Here's how the part is built. I have some questions about the finished solid (model axes, mm). Round coordinates to 2 decimals unless told otherwise and drop trailing zeros. Order: outer loops, then holes, each group sorted by start corner. A loop starts at its lowest first (then second) coordinate and runs counter-clockwise, first axis right, second up. Notation, with made-up numbers: (13.25, 47.25) -> (36.25, 47.25) arc R24 cw to (36.25, 62.25) -> close; hole circle Ø6 at (65, 73.5). An arc over 180 degrees is marked (long way). Use a Markdown table: item, result. Add a question column.
(1) If I drill on probe 1 along Z at (x, y) = (-25, 6.25); probe 2 along X at (y, z) = (1.5, 0.75); probe 3 along X at (y, z) = (8, -0.5), over which ranges is the centre line in solid material (lowest first)?
(2) I want a section at B-B, the plane z = 0. Please give me the cut outline in (x, y).
(3) I want a section at A-A, the plane x = -5. Please give me the cut outline in (y, z).
(4) Thinking about a two-plate mould opening in Z: for faces 1 (the face through (-23.35, 4.93, -0.07)), 2 (the face through (-42, 0, 0)), 3 (the face through (-42, 5, -5)), which applies, pulls with the +Z half, pulls with the -Z half, needs draft (parallel to the pull), parting line crosses it, or undercut?
(5) I want a section at C-C, the plane y = 1.5. Please give me the cut outline in (x, z), then the cut area to 3 significant figures.
Autodesk Inventor part; units mm, degrees
ref_plane "YZ Plane" through (0, 0, 0) normal (1, 0, 0) x (0, 1, 0)
ref_plane "XZ Plane" through (0, 0, 0) normal (0, 1, 0) x (-1, 0, 0)
ref_plane "XY Plane" through (0, 0, 0) normal (0, 0, 1) x (1, 0, 0)
sketch "Sketch1" plane through (0, 0, 0) normal (0, 1, 0) x (-1, 0, 0)
  line L0 (85, 5) -> (0, 5)
  line L1 (0, 5) -> (0, -5)
  line L2 (0, -5) -> (85, -5)
  line L3 (85, -5) -> (85, 5)
  line L4 (25, 0) -> (5, 0) construction
  circle A0 centre (25, 0) radius 1.65
  circle A1 centre (5, 0) radius 1.65
  point P0 (0, 0)
  point P1 (0, 0)
  dimension "d0" = 10
  dimension "d1" = 20
  dimension "d2" = 3.3
  dimension "d3" = 5
  dimension "d6" = 85
extrude "Extrusion1" add sketch "Sketch1" along normal blind 10
properties part number "Tope X" material "Polypropylene"
Taken from the geometry:
| question | item | result |
|---|---|---|
| 1 | probe 1 | z = -5 to -1.65, 1.65 to 5 |
| 1 | probe 2 | x = -85 to -26.47, -23.53 to -6.47, -3.53 to 0 |
| 1 | probe 3 | x = -85 to -26.57, -23.43 to -6.57, -3.43 to 0 |
| 2 | outline | (-85, 0) -> (-26.65, 0) -> (-26.65, 10) -> (-85, 10) -> close; (-23.35, 0) -> (-6.65, 0) -> (-6.65, 10) -> (-23.35, 10) -> close; (-3.35, 0) -> (0, 0) -> (0, 10) -> (-3.35, 10) -> close |
| 3 | outline | (0, -5) -> (10, -5) -> (10, -1.65) -> (0, -1.65) -> close; (0, 1.65) -> (10, 1.65) -> (10, 5) -> (0, 5) -> close |
| 4 | face 1 | undercut |
| 4 | face 2 | needs draft |
| 4 | face 3 | pulls with the -Z half |
| 5 | outline | (-85, -5) -> (0, -5) -> (0, 5) -> (-85, 5) -> close; hole circle Ø3.3 at (-25, 0); hole circle Ø3.3 at (-5, 0) |
| 5 | area | 833 mm2 |
